```python
from build123d import *

# Parameters (mm, degrees)
CROQUIS1_R              = 1.75
CROQUIS1_R_2            = 1.5
SALIENTE_EXTRUIR1_DEPTH = 9
REDONDEO1_R             = 1
CROQUIS2_W              = 2
CROQUIS2_H              = 36
CORTAR_EXTRUIR1_DEPTH   = 71.547856098
REDONDEO2_R             = 3


with BuildPart() as part:
    # Croquis1 → Saliente-Extruir1 (new body)
    with BuildSketch(Plane.XY):
        Polygon((0, 36), (0, 0), (10.5, 0), (10.5, -10), (19.5, -10), (19.5, 0), (40.5, 0), (40.5, -10), (49.5, -10), (49.5, 0), (60, 0), (60, 36), align=None)
        with Locations((6.5, 16.5)):
            Circle(CROQUIS1_R, mode=Mode.SUBTRACT)
        with Locations((6.5, 25.5)):
            Circle(CROQUIS1_R, mode=Mode.SUBTRACT)
        with BuildLine():
            Line((10.5, 26.545268253), (10.5, 31))
            Line((10.5, 31), (15.417424305, 31))
            ThreePointArc((15.417424305, 31), (20, 32), (24.582575695, 31))
            Line((24.582575695, 31), (51.5, 31))
            Line((51.5, 31), (51.5, 11))
            Line((51.5, 11), (24.582575695, 11))
            ThreePointArc((24.582575695, 11), (20, 10), (15.417424305, 11))
            Line((15.417424305, 11), (10.5, 11))
            Line((10.5, 11), (10.5, 15.454731747))
            ThreePointArc((10.5, 15.454731747), (9, 21), (10.5, 26.545268253))
        make_face(mode=Mode.SUBTRACT)
        with Locations((55.5, 16.5)):
            Circle(CROQUIS1_R, mode=Mode.SUBTRACT)
        with Locations((55.5, 25.5)):
            Circle(CROQUIS1_R, mode=Mode.SUBTRACT)
        with Locations((15, -5)):
            Circle(CROQUIS1_R_2, mode=Mode.SUBTRACT)
        with Locations((45, -5)):
            Circle(CROQUIS1_R_2, mode=Mode.SUBTRACT)
    extrude(amount=SALIENTE_EXTRUIR1_DEPTH)

    # Redondeo1
    redondeo1_edges = [part.edges().sort_by_distance(p)[0] for p in [
        (45, -10, 0),
        (15, -10, 0),
        (49.5, -10, 4.5),
        (40.5, -10, 4.5),
        (19.5, -10, 4.5),
        (10.5, -10, 4.5),
        (15, -10, 9),
        (45, -10, 9),
    ]]
    fillet(redondeo1_edges, radius=REDONDEO1_R)

    # Croquis2 → Cortar-Extruir1 (cut, through all)
    with BuildSketch(Plane.ZY):
        with Locations((1, 18)):
            Rectangle(CROQUIS2_W, CROQUIS2_H)
    extrude(amount=-CORTAR_EXTRUIR1_DEPTH, mode=Mode.SUBTRACT)

    # Redondeo2
    # the kernel refuses this fillet: 3 mm, written as the material it adds along each edge
    with BuildSketch(Plane(origin=(10.5, 0, 2), x_dir=(0, 0, -1), z_dir=(1, 0, 0))) as redondeo2_piece_1:
        with BuildLine():
            CenterArc((3, 2.828427125), REDONDEO2_R, 180, 70.528779366)
            Line((0, 2.828427125), (0, 0))
            Line((0, 0), (2, 0))
        make_face()
    extrude(amount=9)
    with BuildSketch(Plane(origin=(40.5, 0, 2), x_dir=(0, 1, 0), z_dir=(1, 0, 0))) as redondeo2_piece_2:
        with BuildLine():
            CenterArc((2.828427125, -3), REDONDEO2_R, 90, 70.528779366)
            Line((0, -2), (0, 0))
            Line((0, 0), (2.828427125, 0))
        make_face()
    extrude(amount=9)


solid = part.part
```
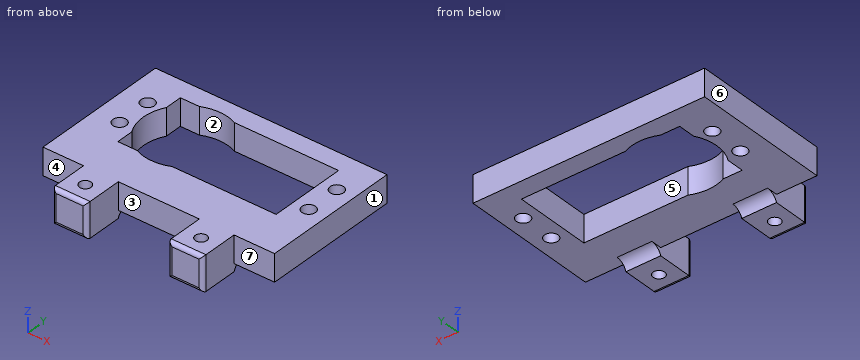
Geometry check sheet. Reference: the model listing, model coordinates, mm. Face numbers are marked on the shaded views. A direction names the side the tool comes from. Coordinates: 2 decimals unless noted, no trailing zeros. Order: outer loops, then holes, each group sorted by start corner. A loop starts at its lowest first (then second) coordinate and runs counter-clockwise, first axis right, second up. Notation, with made-up numbers: (11, 49) - (17, 49) arc R20 cw to (17, 53) - close; hole circle Ø11 at (44.5, 87.25). An arc over 180 degrees is marked (long way). Answer in a Markdown table with one row per item. Add a question column.
1. Section check D-D (z = 6.5). Give the number of separate pieces and of enclosed holes in the cut face, plus the area to 3 significant figures.
2. Section check A-A (x = 6.5). Enter the section's corners in (y, z).
3. Material ranges on L1, parallel to Y at x = 55.5, z = 5; L2, parallel to X at y = -3, z = 6.5; L3, parallel to X at y = 13.5, z = 8.25, recorded low to high. Write a range as [from, to].
4. Access from +Z, -Z, +X, -X, +Y, -Y to the whole of each face (thin tool, end or side, straight path). Record for the marked faces 1, 2, 3 and 4.
5. Section check C-C (x = 38.5). Enter the section's corners in (y, z).
6. Draft check along Y on the marked faces 5, 6 and 7. Enter one of: +Y half, -Y half, draft (parallel to the pull), parting line (faces both ways), or undercut.
7. Gauge pin test, flat ends, axial feed: pin 1 Ø2.5 at (y, z) = (-3.5, 5) entering from -X; pin 2 Ø3.5 at (x, y) = (15, -5) entering from -Z. Record the tip position at first contact, or that the pin passes through.
8. Section check B-B (y = -5). Enter the section's corners in (x, z).
Data:
| question | item | result |
|---|---|---|
| 1 | separate pieces | 1 |
| 1 | enclosed holes | 7 |
| 1 | area | 1,440 mm² |
| 2 | outline | (0, 2) - (14.75, 2) - (14.75, 9) - (0, 9) - close; (18.25, 2) - (23.75, 2) - (23.75, 9) - (18.25, 9) - close; (27.25, 2) - (36, 2) - (36, 9) - (27.25, 9) - close |
| 3 | L1 | y = [0, 14.75], [18.25, 23.75], [27.25, 36] |
| 3 | L2 | x = [10.5, 19.5], [40.5, 49.5] |
| 3 | L3 | x = [0, 10.5], [51.5, 60] |
| 4 | face 1 | +Z, -Z, +X, +Y, -Y |
| 4 | face 2 | +Z, -Z |
| 4 | face 3 | +Z, -Z, -Y |
| 4 | face 4 | +Z, -Z, -X, -Y |
| 5 | outline | (0, 2) - (11, 2) - (11, 9) - (0, 9) - close; (31, 2) - (36, 2) - (36, 9) - (31, 9) - close |
| 6 | face 5 | undercut |
| 6 | face 6 | draft |
| 6 | face 7 | -Y half |
| 7 | pin 1 | stops at x = 10.5 |
| 7 | pin 2 | stops at z = 0 |
| 8 | outline | (10.5, 0) - (13.5, 0) - (13.5, 9) - (10.5, 9) - close; (16.5, 0) - (19.5, 0) - (19.5, 9) - (16.5, 9) - close; (40.5, 0) - (43.5, 0) - (43.5, 9) - (40.5, 9) - close; (46.5, 0) - (49.5, 0) - (49.5, 9) - (46.5, 9) - close |
